Build history of the part. All positions in model axes, mm. Face numbers are marked on the shaded views. A direction names the side the tool comes from. Round coordinates to 2 decimals unless told otherwise and drop trailing zeros. Write each loop counter-clockwise with the first axis right and the second up, starting at its lowest first coordinate (ties: lowest second). Pieces come first, ordered by that corner, then holes. Notation, with made-up numbers: (36.5, 81) - (53.5, 81) arc R12 ccw to (53.5, 103) - close; hole circle Ø11 at (45, 59). An arc over 180 degrees is marked (long way). Write each question's results on one line, items separated by ' | '.
from build123d import *

# Parameters (mm, degrees)
SKETCH1_R           = 9.525
BOSS_EXTRUDE1_DEPTH = 9.525
BOSS_EXTRUDE2_START = 9.525
SKETCH1_4_R         = 9.525
SKETCH1_4_R_2       = 2.413
BOSS_EXTRUDE2_DEPTH = 3.9751
BOSS_EXTRUDE3_START = -9.525
SKETCH1_5_R         = 9.525
SKETCH1_5_R_2       = 2.413
BOSS_EXTRUDE3_DEPTH = 3.9751


with BuildPart() as part:
    # Sketch1 → Boss-Extrude1 (new body, symmetric)
    with BuildSketch(Plane(origin=(0, 0, 0), x_dir=(0, 0, -1), z_dir=(1, 0, 0))):
        Polygon((42.418, 23.552715039), (42.418, 0), (70.358, 0), (70.358, 25.4), (48.514, 25.4), align=None)
        with Locations((57.658, 12.7)):
            Circle(SKETCH1_R, mode=Mode.SUBTRACT)
    extrude(amount=BOSS_EXTRUDE1_DEPTH, both=True)

    # Sketch1<4> → Boss-Extrude2 (add)
    with BuildSketch(Plane(origin=(0, 0, 0), x_dir=(0, 0, -1), z_dir=(1, 0, 0)).offset(BOSS_EXTRUDE2_START)):
        with BuildLine():
            Line((0, 0), (70.358, 0))
            Line((70.358, 0), (70.358, 25.4))
            Line((70.358, 25.4), (48.514, 25.4))
            Line((48.514, 25.4), (17.332880156, 15.95111323))
            ThreePointArc((17.332880156, 15.95111323), (11.05930066, 15.346935831), (5.039023234, 17.212167653))
            Line((5.039023234, 17.212167653), (-7.62, 24.106033067))
            Line((-7.62, 24.106033067), (-16.002, 8.71438754))
            Line((-16.002, 8.71438754), (0, 0))
        make_face()
        with Locations((57.658, 12.7)):
            Circle(SKETCH1_4_R, mode=Mode.SUBTRACT)
        with Locations((-3.556, 12.7)):
            Circle(SKETCH1_4_R_2, mode=Mode.SUBTRACT)
    extrude(amount=-BOSS_EXTRUDE2_DEPTH)

    # Sketch1<5> → Boss-Extrude3 (add)
    with BuildSketch(Plane(origin=(0, 0, 0), x_dir=(0, 0, -1), z_dir=(1, 0, 0)).offset(BOSS_EXTRUDE3_START)):
        with BuildLine():
            Line((0, 0), (70.358, 0))
            Line((70.358, 0), (70.358, 25.4))
            Line((70.358, 25.4), (48.514, 25.4))
            Line((48.514, 25.4), (17.332880156, 15.95111323))
            ThreePointArc((17.332880156, 15.95111323), (11.05930066, 15.346935831), (5.039023234, 17.212167653))
            Line((5.039023234, 17.212167653), (-7.62, 24.106033067))
            Line((-7.62, 24.106033067), (-16.002, 8.71438754))
            Line((-16.002, 8.71438754), (0, 0))
        make_face()
        with Locations((57.658, 12.7)):
            Circle(SKETCH1_5_R, mode=Mode.SUBTRACT)
        with Locations((-3.556, 12.7)):
            Circle(SKETCH1_5_R_2, mode=Mode.SUBTRACT)
    extrude(amount=BOSS_EXTRUDE3_DEPTH)


solid = part.part
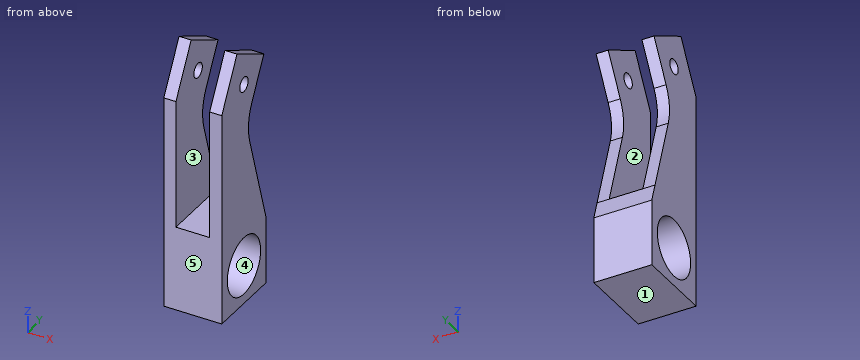
(1) Flat gauge pins, fed straight in: pin 1 Ø8 at (x, z) = (4, 2.5) entering from +Y; pin 2 Ø3.5 at (x, y) = (1, 14) entering from +Z; pin 3 Ø5.5 at (y, z) = (12.7, 3.556) entering from -X (3 decimals). Where does each tip first touch, or does it go through?
Worked answers:
pin 1: stops at y = 23.33 | pin 2: stops at z = -42.42 | pin 3: stops at x = -9.525
(2) Slice it at B-B, the plane x = -6.5. Write the cut outline in (y, z) (3 decimals).
Worked answers:
outline: (0, -70.358) - (25.4, -70.358) - (25.4, -48.514) - (15.951, -17.333) arc R16.002 cw to (17.212, -5.039) - (24.106, 7.62) - (8.714, 16.002) - (0, 0) - close; hole circle Ø19.05 at (12.7, -57.658); hole circle Ø4.826 at (12.7, 3.556)
(3) Tool access for the marked faces 1 and 2: list every direction of +Z, -Z, +X, -X, +Y, -Y with a clear straight run to the whole face (end or side of a thin tool).
Worked answers:
face 1: -Z, +X, -X, +Y, -Y | face 2: +Z, +Y, -Y
(4) Drill centre lines: probe 1 along X at (y, z) = (9.75, -23) (3 decimals); probe 2 along Z at (x, y) = (3, 13); probe 3 along Z at (x, y) = (-0.5, 2). Where is each one in solid material? Low to high. Write a range as [from, to].
Worked answers:
probe 1: x = [-9.525, -5.55], [5.55, 9.525] | probe 2: z = [-70.36, -67.18], [-48.14, -42.42] | probe 3: z = [-70.36, -42.42]
(5) Slice it at C-C, the plane y = 12.7. Write the cut outline in (x, z) (3 decimals), and give its area (3 significant figures).
Worked answers:
outline: (-9.525, -70.358) - (9.525, -70.358) - (9.525, -67.183) - (-9.525, -67.183) - close; (-9.525, -48.133) - (9.525, -48.133) - (9.525, 1.143) - (5.55, 1.143) - (5.55, -42.418) - (-5.55, -42.418) - (-5.55, 1.143) - (-9.525, 1.143) - close; (-9.525, 5.969) - (-5.55, 5.969) - (-5.55, 13.832) - (-9.525, 13.832) - close; (5.55, 5.969) - (9.525, 5.969) - (9.525, 13.832) - (5.55, 13.832) - close | area: 578 mm2
(6) Slice it at D-D, the plane x = 0. Write the cut outline in (y, z) (3 decimals).
Worked answers:
outline: (0, -70.358) - (25.4, -70.358) - (25.4, -48.514) - (23.553, -42.418) - (0, -42.418) - close; hole circle Ø19.05 at (12.7, -57.658)
(7) Two-plate mould, pull along Y, no slides. Class the marked faces 3, 4 and 5: released by +Y, released by -Y, zero draft, split by the parting line, or undercut.
Worked answers:
face 3: zero draft | face 4: undercut | face 5: released by -Y
(8) Slice it at A-A, the plane z = -29.5. Write the cut outline in (x, y) (3 decimals), and give its area (3 significant figures).
Worked answers:
outline: (-9.525, 0) - (-5.55, 0) - (-5.55, 19.638) - (-9.525, 19.638) - close; (5.55, 0) - (9.525, 0) - (9.525, 19.638) - (5.55, 19.638) - close | area: 156 mm2
